Geometry: final body of the model. Coordinates: model frame, mm. A direction names the side the tool comes from. Give positions to 0.01 mm unless a question says otherwise; leave off trailing zeros. Write each loop counter-clockwise with the first axis right and the second up, starting at its lowest first coordinate (ties: lowest second). Pieces come first, ordered by that corner, then holes.
from build123d import *

# Parameters (mm, degrees)
SKETCH2_W          = 1.25
SKETCH2_H          = 11
SKETCH4_W          = 1.25
SKETCH4_H          = 11
SKETCH6_R          = 3
CUT_EXTRUDE1_DEPTH = 24.414739023


with BuildPart() as part:
    # Sketch1 → Revolve1 (revolve)
    with BuildSketch(Plane.XY, mode=Mode.PRIVATE) as revolve1_sk:
        Polygon((0, 2.5), (0, 6), (6.3, 6), (6.3, 11), (7.9, 11), (7.9, 9.325), (15.9, 9.325), (15.9, 11), (17.5, 11), (17.5, 2.5), align=None)
    revolve(revolve1_sk.sketch.rotate(Axis((0, 0, 0), (-1, 0, 0)), 90), axis=Axis((0, 0, 0), (-1, 0, 0)))

    # Sketch2 → M3x0.5 Tapped Hole1 (revolve, cut)
    with BuildSketch(Plane(origin=(3.15, 0, 0), x_dir=(0, 0, -1), z_dir=(1, 0, 0))):
        with Locations((0.625, 5.5)):
            Rectangle(SKETCH2_W, SKETCH2_H)
    revolve(axis=Axis((3.15, -6.35, 0), (0, 1, 0)), mode=Mode.SUBTRACT)

    # Sketch4 → M3x0.5 Tapped Hole2 (revolve, cut)
    with BuildSketch(Plane.YZ.offset(3.15)):
        with Locations((0.625, 5.5)):
            Rectangle(SKETCH4_W, SKETCH4_H)
    revolve(axis=Axis((3.15, 0, -6.35), (0, 0, 1)), mode=Mode.SUBTRACT)

    # Sketch6 → Cut-Extrude1 (cut, through all)
    with BuildSketch(Plane(origin=(17.5, 0, 0), x_dir=(0, 0, -1), z_dir=(1, 0, 0))):
        Circle(SKETCH6_R)
    extrude(amount=-CUT_EXTRUDE1_DEPTH, mode=Mode.SUBTRACT)


solid = part.part
Q1. Section D-D on y = -3.75. Output: boundary loops of the cut face in (x, z).
Filled sheet:
outline: (0, -4.68) - (6.3, -4.68) - (6.3, -10.34) - (7.9, -10.34) - (7.9, -8.54) - (15.9, -8.54) - (15.9, -10.34) - (17.5, -10.34) - (17.5, 10.34) - (15.9, 10.34) - (15.9, 8.54) - (7.9, 8.54) - (7.9, 10.34) - (6.3, 10.34) - (6.3, 4.68) - (0, 4.68) - close
Q2. Pull-direction query (X, two-part tool) for faces 1 (the cylindrical face through (11.956, 9.103, 2.021)), 2 (the cylindrical face through (7.11, 10.74, 2.38)), 3 (the flat face through (6.3, 5, 5)), 4 (the flat face through (17.5, 2.3, -2.3)); classes: released by +X, released by -X, zero draft, split by the parting line, or undercut.
Filled sheet:
face 1: undercut
face 2: zero draft
face 3: released by -X
face 4: released by +X
Q3. Pin query (flat end, axial travel): P1, Ø4, axis at x = 11, y = -6, coming from the -Z side; P2, Ø1.5, axis at x = 3.15, y = 0, coming from the -Z side; P3, Ø1, axis at x = 6.5, z = 4, coming from the +Y side; P4, Ø6.5, axis at y = -5, z = 3, coming from the -X side. Return the tip coordinate at first contact, or that it passes through.
Filled sheet:
P1: stops at z = -8.42
P2: stops at z = -6
P3: stops at y = 10.43
P4: stops at x = 0
Q4. Section A-A on z = 0. Output: boundary loops of the cut face in (x, y) (3 decimals), plus the area to 3 significant figures.
Filled sheet:
outline: (0, -6) - (6.3, -6) - (6.3, -11) - (7.9, -11) - (7.9, -9.325) - (15.9, -9.325) - (15.9, -11) - (17.5, -11) - (17.5, -3) - (0, -3) - close; (0, 3) - (1.9, 3) - (1.9, 6) - (0, 6) - close; (4.4, 3) - (17.5, 3) - (17.5, 11) - (15.9, 11) - (15.9, 9.325) - (7.9, 9.325) - (7.9, 11) - (6.3, 11) - (6.3, 6) - (4.4, 6) - close
area: 183 mm2
Q5. Section B-B on x = 3.15. Output: boundary loops of the cut face in (y, z).
Filled sheet:
outline: (-1.25, 2.73) - (-1.25, 5.87) arc R6 ccw (long way) to (5.87, -1.25) - (2.73, -1.25) arc R3 cw (long way) to start; (1.25, 2.73) arc R3 cw to (2.73, 1.25) - (5.87, 1.25) arc R6 ccw to (1.25, 5.87) - close
Q6. Ray query, line 1 along Y through (x, z) = (14.25, 0) (3 decimals); line 2 along X through (y, z) = (4.25, 0); line 3 along X through (y, z) = (4.75, 8.25). Return the intervals inside material, ascending.
Filled sheet:
line 1: y = -9.325 to -3, 3 to 9.325
line 2: x = 0 to 1.9, 4.4 to 17.5
line 3: x = 6.3 to 7.9, 15.9 to 17.5
Q7. Section C-C on y = 3.5. Output: boundary loops of the cut face in (x, z), plus the area to 3 significant figures.
Filled sheet:
outline: (0, -4.87) - (6.3, -4.87) - (6.3, -10.43) - (7.9, -10.43) - (7.9, -8.64) - (15.9, -8.64) - (15.9, -10.43) - (17.5, -10.43) - (17.5, 10.43) - (15.9, 10.43) - (15.9, 8.64) - (7.9, 8.64) - (7.9, 10.43) - (6.3, 10.43) - (6.3, 4.87) - (0, 4.87) - close; hole circle Ø2.5 at (3.15, 0)
area: 262 mm2
Q8. Access query for faces 5 (the cylindrical face through (1.91, 4.39, 0.16)), 6 (the flat face through (7.9, -4.9, 8.2)), 7 (the cylindrical face through (1.91, -0.16, 4.39)), 8 (the cylindrical face through (3.194, -1.802, -5.723)). Directions: +Z, -Z, +X, -X, +Y, -Y. A direction counts if a zero-diameter tool reaches every point of the face in a straight line with its end or side. Return the directions, or none.
Filled sheet:
face 5: +Y
face 6: none
face 7: +Z
face 8: -X
